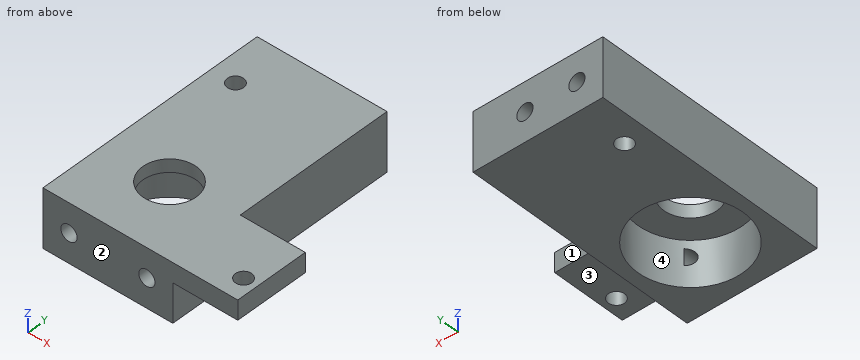
Autodesk Inventor part; units mm, degrees
ref_plane "Plano de trabajo1" through (-47.2143, 36.5, -75.5) normal (0, -1, 0) x (1, 0, 0)
ref_plane "YZ Plane" through (0, 0, 0) normal (1, 0, 0) x (0, 1, 0)
ref_plane "XZ Plane" through (0, 0, 0) normal (0, 1, 0) x (-1, 0, 0)
ref_plane "Plano de trabajo1" through (-47.2143, 36.5, -75.5) normal (0, -1, 0) x (1, 0, 0)
sketch "Boceto1" plane through (0, 0, 0) normal (0, 1, 0) x (-1, 0, 0)
  line L0 (0, 0) -> (20, 0)
  line L1 (20, 0) -> (20, -9)
  line L2 (20, -9) -> (0, -9)
  line L3 (0, -9) -> (0, 0)
  line L4 (0, 0) -> (-10, 0)
  line L5 (-10, 0) -> (-10, -3)
  line L6 (-10, -3) -> (0, -3)
  line L7 (0, -3) -> (0, 0)
  dimension "d0" = 20
  dimension "d1" = 9
  dimension "d25" = 10
  dimension "d26" = 3
extrude "Extrusión1" add sketch "Boceto1" along normal up to surface (36.5 mm away)
sketch "Boceto2" plane through (0, 0, -9) normal (0, 0, -1) x (-1, 0, 0)
  circle A0 centre (10, 10.5) radius 4.5
  point P0 (0, 0)
hole "Agujero1" at (-10, 10.5, -9) direction (0, 0, 1) diameter 16.2 depth 7
sketch "Boceto3" plane through (0, 0, -9) normal (0, 0, -1) x (-1, 0, 0)
  circle A0 centre (10, 10.5) radius 8.1
  point P0 (0, 0)
hole "Agujero2" at (-10, 10.5, -9) direction (0, 0, 1) diameter 8.2 end through all
sketch "Boceto4" plane through (0, 0, 0) normal (0, -1, 0) x (1, 0, 0)
  circle A0 centre (-4, -4.5) radius 1.25
  circle A1 centre (-16, -4.5) radius 1.25
  point P0 (0, 0)
hole "Agujero3" at (-16, 0, -4.5) at (-4, 0, -4.5) direction (0, 1, 0) diameter 2.5 depth 5
sketch "Boceto6" plane through (-20, 36.5, 0) normal (0, 1, 0) x (1, 0, 0)
  line L0 (30, 0) -> (30, 3)
  line L1 (30, 3) -> (20, 3)
  line L2 (20, 3) -> (20, 0)
  line L3 (20, 0) -> (30, 0)
  line L4 (30, 0) -> (30, 3)
extrude "Extrusión2" cut sketch "Boceto6" against normal blind 25
sketch "Boceto7" plane through (-20, 0, 0) normal (0, 0, 1) x (1, 0, 0)
  circle A0 centre (3.7217, 28.6888) radius 2.1
  circle A1 centre (27.863, 3.3471) radius 2.1
  circle A2 centre (3.7217, 28.6888) radius 1.25
  circle A3 centre (27.863, 3.3471) radius 1.25
  point P0 (20, 0)
  dimension "d31" = 2.5
  dimension "d32" = 2.5
extrude "Extrusión3" cut sketch "Boceto7" against normal through all contours A2 | A3
sketch "Boceto8" plane through (-20, 36.5, -9) normal (0, 1, 0) x (1, 0, 0)
  line L0 (0, 0) -> (0, -9)
  line L1 (0, -4.5) -> (4, -4.5)
  line L2 (4, -4.5) -> (12, -4.5)
  circle A0 centre (4, -4.5) radius 1.25
  circle A1 centre (12, -4.5) radius 1.25
  point P0 (20, -9)
  dimension "d33" = 4
  dimension "d34" = 8
  dimension "d35" = 2.5
extrude "Extrusión4" cut sketch "Boceto8" against normal blind 10
properties part number "Soporte mecanismo 2"
Here's how the part is built. I have some questions about the finished solid (model axes, mm). Face numbers are marked on the shaded views. A direction names the side the tool comes from. Coordinates: 2 decimals unless noted, no trailing zeros. Order: outer loops, then holes, each group sorted by start corner. A loop starts at its lowest first (then second) coordinate and runs counter-clockwise, first axis right, second up. Notation, with made-up numbers: M 26,-4.5 L 52,-4.5 A21 cw 52,32.5 Z; hole C 32.25,31 d7. An arc over 180 degrees is marked long. Answer as a JSON object with one key per item and string values. Group by question number.
(1) For pin 1 (1 mm diameter, centred on y = 28, z = -4, fed in from +X); pin 2 (2 mm diameter, centred on x = -4, z = -4.5, fed in from -Y); pin 3 (8 mm diameter, centred on x = -9, y = 10.5, fed in from -Z), each with a flat end and sliding along its axis, tell me the tip position at first contact or that it passes through.
(2) Which directions (+Z, -Z, +X, -X, +Y, -Y) give clear straight access to the entire face, cutting with the end or side of a thin tool? Please do the marked faces 1, 2, 3 and 4.
(3) Suppose I cut it at C-C, the plane y = 28. Please give me the cut outline in (x, z), then the cut area to 3 significant figures.
(4) Suppose I cut it at A-A, the plane y = 10.5. Please give me the cut outline in (x, z).
(5) Suppose I cut it at D-D, the plane x = -13.25. Please give me the cut outline in (y, z), then the cut area to 3 significant figures.
(6) Suppose I cut it at B-B, the plane x = -10. Please give me the cut outline in (y, z), then the cut area to 3 significant figures.
(7) I need wall thicknesses on probe 1 along X at (y, z) = (29.75, -4.5); probe 2 along X at (y, z) = (1.5, -4.5); probe 3 along Z at (x, y) = (-4, 1.2). Which ranges of each line are inside material? Lowest first, please.
Values found:
{
 "1": {"pin 1": "stops at x = 0", "pin 2": "stops at y = 5", "pin 3": "stops at z = -2"},
 "2": {"face 1": "+Z, -Z, +X, +Y", "face 2": "+Z, -Z, +X, -X, -Y", "face 3": "-Z, +X, +Y, -Y", "face 4": "-Z"},
 "3": {"outline": "M -20,-9 L -17.32,-9 L -17.32,0 L -20,0 Z; M -15.24,-9 L 0,-9 L 0,0 L -15.24,0 L -15.24,-3.51 A1.25 cw -15.24,-5.49 Z; hole C -8,-4.5 d2.5", "area": "156 mm^2"},
 "4": {"outline": "M -20,-9 L -18.1,-9 L -18.1,-2 L -14.1,-2 L -14.1,0 L -20,0 Z; M -5.9,-2 L -1.9,-2 L -1.9,-9 L 0,-9 L 0,-3 L 10,-3 L 10,0 L -5.9,0 Z"},
 "5": {"outline": "M 0,-9 L 3.08,-9 L 3.08,-2 L 8,-2 L 8,0 L 0,0 Z; M 13,-2 L 17.92,-2 L 17.92,-9 L 36.5,-9 L 36.5,0 L 13,0 Z", "area": "215 mm^2"},
 "6": {"outline": "M 0,-9 L 2.4,-9 L 2.4,-2 L 6.4,-2 L 6.4,0 L 0,0 Z; M 14.6,-2 L 18.6,-2 L 18.6,-9 L 36.5,-9 L 36.5,0 L 14.6,0 Z", "area": "199 mm^2"},
 "7": {"probe 1": "x = -20 to -17.25, -14.75 to -9.25, -6.75 to 0", "probe 2": "x = -20 to -17.25, -14.75 to -5.25, -2.75 to 0", "probe 3": "z = -9 to -5.75, -3.25 to 0"}
}
